from build123d import *

# Parameters (mm, degrees)
F1_DEPTH = 158.75
F2_R     = 50


with BuildPart() as f1:
    # F0 (on Front) → F1 (new body, symmetric)
    with BuildSketch(Plane.XZ):
        with BuildLine():
            Line((-200.025, -9.525), (250.825, -9.525))
            Line((250.825, -9.525), (250.825, 9.525))
            Line((250.825, 9.525), (-191.671143, 9.525))
            ThreePointArc((-191.671143, 9.525), (-200.066769, 8.826432), (-208.231493, 6.749939))
            Line((-208.231493, 6.749939), (-250.825, -7.9375))
            Line((-250.825, -7.9375), (-250.825, -9.525))
            Line((-250.825, -9.525), (-200.025, -9.525))
        make_face()
    extrude(amount=F1_DEPTH, both=True)

    # F2
    f2_edges = [f1.edges().sort_by_distance(p)[0] for p in [
        (-250.825, -158.75, -8.73125),
        (250.825, -158.75, 0),
        (250.825, 158.75, 0),
    ]]
    fillet(f2_edges, radius=F2_R)


solid = f1.part
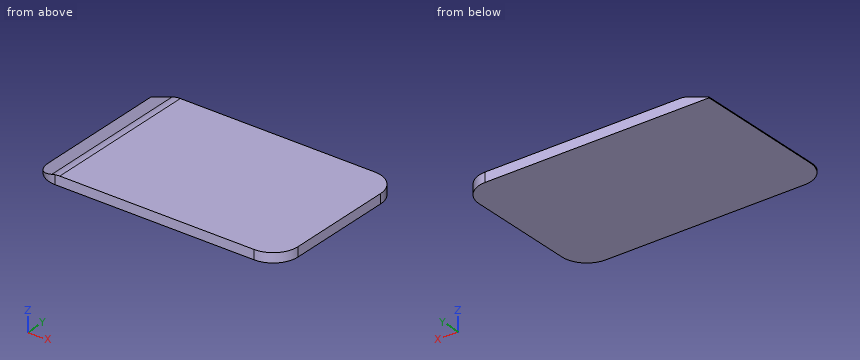
Work out the finished part from the listing and answer in its coordinate system (mm). Round coordinates to 2 decimals unless told otherwise and drop trailing zeros. Write each loop counter-clockwise with the first axis right and the second up, starting at its lowest first coordinate (ties: lowest second). Pieces come first, ordered by that corner, then holes.
1) A cutting plane is placed at B-B (z = 1.5). Give the vertices of the cut face in (x, y) (3 decimals).
2) A cutting plane is placed at A-A (y = 36.5). Give the vertices of the cut face in (x, z) (1 decimal), plus the area to 3 significant figures.
3) A cutting plane is placed at C-C (y = 138). Give the vertices of the cut face in (x, z) (1 decimal), plus the area to 3 significant figures.
4) Straight lines are drawn through the part: line 1 (X direction, y = 110, z = -8.5) (3 decimals); line 2 (Y direction, x = 221, z = -5); line 3 (X direction, y = -144, z = -5.75). For each, find the intervals that lie inside material, in ascending order.
5) Given pin 1 Ø10 at (y, z) = (-121.5, 2.5) entering from +X, flat-ended and moving along its own axis, determine where the tip first touches the part or whether it passes through.
Completed:
1. outline: (-223.456, -153.335) arc R50 ccw to (-200.825, -158.75) - (200.825, -158.75) arc R50 ccw to (250.825, -108.75) - (250.825, 108.75) arc R50 ccw to (200.825, 158.75) - (-223.456, 158.75) - close
2. outline: (-250.8, -9.5) - (250.8, -9.5) - (250.8, 9.5) - (-191.7, 9.5) arc R50.8 ccw to (-208.2, 6.7) - (-250.8, -7.9) - close
2. area: 9,110 mm2
3. outline: (-250.8, -9.5) - (241.4, -9.5) - (241.4, 9.5) - (-191.7, 9.5) arc R50.8 ccw to (-208.2, 6.7) - (-250.8, -7.9) - close
3. area: 8,930 mm2
4. line 1: x = -250.825 to 250.809
4. line 2: y = -154.5 to 154.5
4. line 3: x = -236.29 to 236.29
5. pin 1: stops at x = 250.22
